```python
from build123d import *

# Parameters (mm, degrees)
F0_W     = 800
F0_H     = 520
F1_DEPTH = 60
F2_W     = 400
F2_H     = 200
F3_DEPTH = 30
F4_W     = 80
F4_H     = 30
F5_DEPTH = 200
F6_W     = 730
F6_H     = 450
F7_DEPTH = 5


with BuildPart() as f1:
    # F0 (on Top) → F1 (new body)
    with BuildSketch(Plane.XY):
        with Locations((-400, -260)):
            Rectangle(F0_W, F0_H)
    extrude(amount=F1_DEPTH)

    # F2 (on face) → F3 (join)
    with BuildSketch(Plane(origin=(0, 0, 0), x_dir=(1, 0, 0), z_dir=(0, 0, -1))):
        with Locations((-400, 260)):
            Rectangle(F2_W, F2_H)
    extrude(amount=F3_DEPTH)

    # F4 (on face) → F5 (join)
    with BuildSketch(Plane.XZ.offset(360)):
        with Locations((-400, -15)):
            Rectangle(F4_W, F4_H)
    extrude(amount=F5_DEPTH)

    # F6 (on face) → F7 (cut)
    with BuildSketch(Plane.XY.offset(60)):
        with Locations((-400, -260)):
            Rectangle(F6_W, F6_H)
    extrude(amount=-F7_DEPTH, mode=Mode.SUBTRACT)


solid = f1.part
```
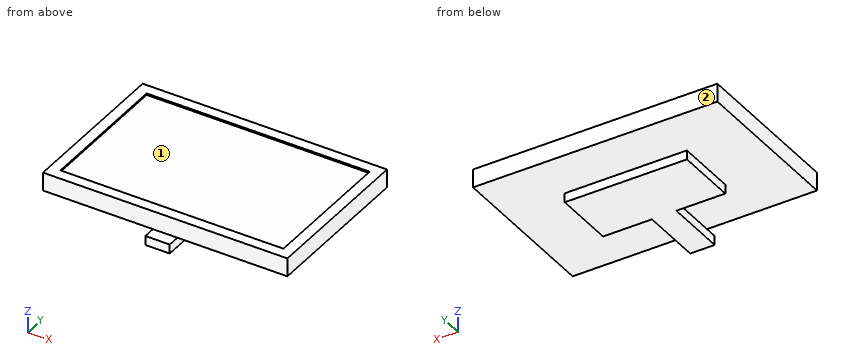
Check sheet for the modelled part. Datum: model origin and axes. Units: mm. Face numbers are marked on the shaded views. Coordinates: 2 decimals unless noted, no trailing zeros. Loops run counter-clockwise (first coordinate to the right, second up) from the corner with the lowest first, then second, coordinate; pieces in that order, holes last.
1) Sectioned sample at A-A (z = -22). Record the boundary of the cut face in (x, y), and give its area (3 significant figures).
2) Sectioned sample at B-B (x = -687). Record the boundary of the cut face in (y, z).
3) Sectioned sample at D-D (x = -567). Record the boundary of the cut face in (y, z).
4) Material ranges on probe 1 along Z at (x, y) = (-739, -61); probe 2 along Z at (x, y) = (-383.5, -531); probe 3 along X at (y, z) = (-247, -24), recorded low to high.
5) Release check for a two-part mould opening along X. For the marked faces 1 and 2 record: released by +X, released by -X, zero draft, split by the parting line, or undercut.
6) Sectioned sample at C-C (y = -185). Record the boundary of the cut face in (x, z).
7) Gauge pin test, flat ends, axial feed: pin 1 (24 mm diameter, centred on x = -271, z = -17.5, fed in from -Y); pin 2 (15 mm diameter, centred on y = -434.5, z = -8, fed in from -X); pin 3 (6 mm diameter, centred on x = -599, y = -121.5, fed in from +Z). Record the tip position at first contact, or that the pin passes through.
Check sheet entries:
1. outline: (-600, -360) - (-440, -360) - (-440, -560) - (-360, -560) - (-360, -360) - (-200, -360) - (-200, -160) - (-600, -160) - close
1. area: 96,000 mm2
2. outline: (-520, 0) - (0, 0) - (0, 60) - (-35, 60) - (-35, 55) - (-485, 55) - (-485, 60) - (-520, 60) - close
3. outline: (-520, 0) - (-360, 0) - (-360, -30) - (-160, -30) - (-160, 0) - (0, 0) - (0, 60) - (-35, 60) - (-35, 55) - (-485, 55) - (-485, 60) - (-520, 60) - close
4. probe 1: z = 0 to 55
4. probe 2: z = -30 to 0
4. probe 3: x = -600 to -200
5. face 1: undercut
5. face 2: zero draft
6. outline: (-800, 0) - (-600, 0) - (-600, -30) - (-200, -30) - (-200, 0) - (0, 0) - (0, 60) - (-35, 60) - (-35, 55) - (-765, 55) - (-765, 60) - (-800, 60) - close
7. pin 1: stops at y = -360
7. pin 2: stops at x = -440
7. pin 3: stops at z = 55
